Design review of the part built by this model. Coordinates are the model's own, in mm. Face numbers are marked on the shaded views. Round coordinates to 2 decimals unless told otherwise and drop trailing zeros. Loops run counter-clockwise (first coordinate to the right, second up) from the corner with the lowest first, then second, coordinate; pieces in that order, holes last. Notation, with made-up numbers: M 19.25,-22.5 L 30.25,-22.5 A24 ccw 30.25,-11.5 Z; hole C 21.25,-18.75 d11. An arc over 180 degrees is marked long. One line per item, written item: value. Start each with the question number.
Item 1: Mouldability with a two-part tool opening along Y and no side actions: class the marked faces 1 and 2 as released by +Y, released by -Y, zero draft, split by the parting line, or undercut.
Item 2: For line 1 along Y through (x, z) = (-6.5, -2.5); line 2 along X through (y, z) = (22.5, -1.75); line 3 along X through (y, z) = (75, 3.25), list the stretches that pass through material, from the lowest coordinate up.
Item 3: We need section A-A (y = 70). Write out the cut boundary in (x, z), then the cut area to 3 significant figures.
Item 4: Clearance check with flat-ended pins moving along their axes: pin 1 (3 mm diameter, centred on x = -1.5, y = 115, fed in from -Z); pin 2 (4 mm diameter, centred on y = 61.5, z = 5, fed in from -X); pin 3 (2 mm diameter, centred on y = 84, z = -1.5, fed in from +X). State where each tip first meets the part, or that it passes through.
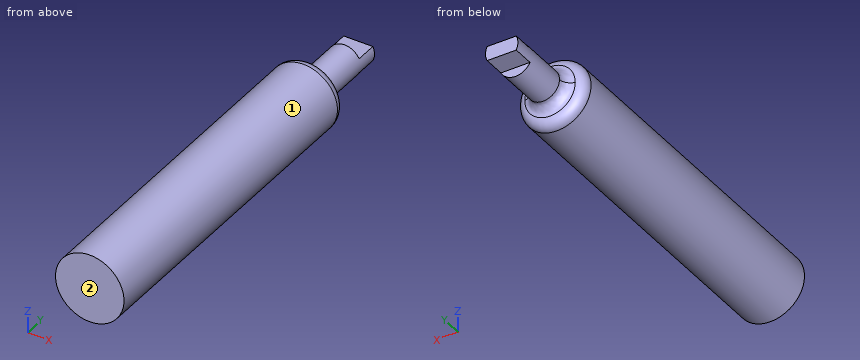
Autodesk Inventor part; units mm, degrees
ref_plane "YZ Plane" through (0, 0, 0) normal (1, 0, 0) x (0, 1, 0)
ref_plane "XZ Plane" through (0, 0, 0) normal (0, 1, 0) x (-1, 0, 0)
ref_plane "XY Plane" through (0, 0, 0) normal (0, 0, 1) x (1, 0, 0)
sketch "Sketch1" plane through (0, 0, 0) normal (0, 1, 0) x (-1, 0, 0)
  circle A0 centre (0, 0) radius 9.5
  dimension "d0" = 19
extrude "Extrusion1" add sketch "Sketch1" along normal blind 96
sketch "Sketch2" plane through (0, 96, 0) normal (0, 1, 0) x (1, 0, 0)
  circle A0 centre (0, 0) radius 4.5
  dimension "d3" = 9
extrude "Extrusion2" add sketch "Sketch2" along normal blind 15
sketch "Sketch3" plane through (0, 111, 0) normal (0, 1, 0) x (1, 0, 0)
  circle A0 centre (0, 0) radius 4.5
  line L0 (-4.5, -2) -> (4.5, -2)
  line L1 (4.5, -2) -> (4.5, 2)
  line L2 (4.5, 2) -> (-4.5, 2)
  line L3 (-4.5, 2) -> (-4.5, -2)
  point P0 (-4.5, 0)
  point P1 (0, 2)
  point P2 (4.0311, 2)
  point P3 (-4.0311, 2)
  point P4 (-4.0311, -2)
  point P5 (4.0311, -2)
  dimension "d6" = 4
extrude "Extrusion3" add sketch "Sketch3" along normal blind 6 contours A0 L0 L2
fillet "Fillet1" radius 3 2 edges at (9.5, 96, 0) (-4.5, 96, 0)
properties part number "Marker" material "PC/ABS Plastic"
A:
1. face 1: zero draft
1. face 2: released by -Y
2. line 1: 0 to 95.96
2. line 2: -9.34 to 9.34
2. line 3: -8.93 to 8.93
3. outline: C 0,0 d19
3. area: 284 mm2
4. pin 1: z = -2
4. pin 2: x = -9.01
4. pin 3: x = 9.49
